```python
from build123d import *

# Parameters (mm, degrees)
F3_T      = -3.175
F5_DEPTH  = 31.75
F7_DEPTH  = 31.75
F9_DEPTH  = 31.75
F10_R     = 12.7
F11_DEPTH = 25.4
F12_W     = 12.7
F12_H     = 6.35
F13_DEPTH = 7.62
F15_DEPTH = 6.35
F16_R     = 6.35
F17_DEPTH = 25.4


with BuildPart() as f2:
    # F0 (on Front) → F2 (revolve)
    with BuildSketch(Plane.XZ):
        Polygon((-34.925, 0), (0, 0), (0, 34.925), (-47.625, 34.925), align=None)
    revolve(axis=Axis((0, 0, 24.3954025209), (0, 0, 1)))

    # F3
    f3_openings = [f2.faces().sort_by_distance(p)[0] for p in [
        (0, 0, 34.925),
    ]]
    offset(amount=F3_T, openings=f3_openings)

    # F4 (on face) → F5 (join)
    with BuildSketch(Plane(origin=(0, 0, 0), x_dir=(1, 0, 0), z_dir=(0, 0, -1))):
        with BuildLine():
            Line((-32.8328621344, 11.90625), (-11.90625, 11.90625))
            Line((-11.90625, 11.90625), (-11.90625, 32.8328621344))
            ThreePointArc((-11.90625, 32.8328621344), (-13.5101727919, 32.2060686227), (-15.08125, 31.5009765474))
            Line((-15.08125, 31.5009765474), (-15.08125, 15.08125))
            Line((-15.08125, 15.08125), (-31.5009765474, 15.08125))
            ThreePointArc((-31.5009765474, 15.08125), (-32.2060686227, 13.5101727919), (-32.8328621344, 11.90625))
        make_face()
        with BuildLine():
            Line((-11.90625, -32.8328621344), (-11.90625, -11.90625))
            Line((-11.90625, -11.90625), (-32.8328621344, -11.90625))
            ThreePointArc((-32.8328621344, -11.90625), (-32.2060686227, -13.5101727919), (-31.5009765474, -15.08125))
            Line((-31.5009765474, -15.08125), (-15.08125, -15.08125))
            Line((-15.08125, -15.08125), (-15.08125, -31.5009765474))
            ThreePointArc((-15.08125, -31.5009765474), (-13.5101727919, -32.2060686227), (-11.90625, -32.8328621344))
        make_face()
        with BuildLine():
            Line((32.8328621344, -11.90625), (11.90625, -11.90625))
            Line((11.90625, -11.90625), (11.90625, -32.8328621344))
            ThreePointArc((11.90625, -32.8328621344), (13.5101727919, -32.2060686227), (15.08125, -31.5009765474))
            Line((15.08125, -31.5009765474), (15.08125, -15.08125))
            Line((15.08125, -15.08125), (31.5009765474, -15.08125))
            ThreePointArc((31.5009765474, -15.08125), (32.2060686227, -13.5101727919), (32.8328621344, -11.90625))
        make_face()
        with BuildLine():
            Line((11.90625, 32.8328621344), (11.90625, 11.90625))
            Line((11.90625, 11.90625), (32.8328621344, 11.90625))
            ThreePointArc((32.8328621344, 11.90625), (32.2060686227, 13.5101727919), (31.5009765474, 15.08125))
            Line((31.5009765474, 15.08125), (15.08125, 15.08125))
            Line((15.08125, 15.08125), (15.08125, 31.5009765474))
            ThreePointArc((15.08125, 31.5009765474), (13.5101727919, 32.2060686227), (11.90625, 32.8328621344))
        make_face()
    extrude(amount=F5_DEPTH)

    # F6 (on face) → F7 (cut, through all)
    with BuildSketch(Plane.XY.offset(34.925)):
        Polygon((15.7154482119, 51.6364726961), (0, 0), (51.6364726961, 15.7154482119), (33.675960454, 33.675960454), align=None)
    extrude(amount=-F7_DEPTH, mode=Mode.SUBTRACT)

    # F8 (on face) → F9 (cut, through all)
    with BuildSketch(Plane.XY.offset(34.925)):
        with BuildLine():
            Line((-27.3165777812, 39.0121161093), (0, 0))
            Line((0, 0), (0, 47.625))
            ThreePointArc((0, 47.625), (-14.3211137014, 45.4207697794), (-27.3165777812, 39.0121161093))
        make_face()
        with BuildLine():
            Line((-39.0121161093, -27.3165777812), (0, 0))
            Line((0, 0), (-39.0121161093, 27.3165777812))
            ThreePointArc((-39.0121161093, 27.3165777812), (-47.625, 0), (-39.0121161093, -27.3165777812))
        make_face()
        with BuildLine():
            Line((27.3165777812, -39.0121161093), (0, 0))
            Line((0, 0), (-27.3165777812, -39.0121161093))
            ThreePointArc((-27.3165777812, -39.0121161093), (0, -47.625), (27.3165777812, -39.0121161093))
        make_face()
        with BuildLine():
            Line((47.625, 0), (0, 0))
            Line((0, 0), (39.0121161093, -27.3165777812))
            ThreePointArc((39.0121161093, -27.3165777812), (45.4207697794, -14.3211137014), (47.625, 0))
        make_face()
    extrude(amount=-F9_DEPTH, mode=Mode.SUBTRACT)

    # F10 (on face) → F11 (cut)
    with BuildSketch(Plane.XY.offset(3.175)):
        Circle(F10_R)
    extrude(amount=-F11_DEPTH, mode=Mode.SUBTRACT)

    # F12 (on face) → F13 (join)
    with BuildSketch(Plane.YZ.offset(15.08125)):
        with Locations((23.2911132737, -15.875)):
            Rectangle(F12_W, F12_H)
    extrude(amount=F13_DEPTH)

    # F14 (on face) → F15 (cut, through all)
    with BuildSketch(Plane(origin=(0, 0, -19.05), x_dir=(1, 0, 0), z_dir=(0, 0, -1))):
        with BuildLine():
            Line((16.1188345795, -28.8882274593), (20.7059307299, -22.1824388165))
            ThreePointArc((20.7059307299, -22.1824388165), (20.8007868478, -19.6961173416), (18.5999628156, -18.5354426503))
            Line((18.5999628156, -18.5354426503), (15.08125, -18.5354426503))
            Line((15.08125, -18.5354426503), (15.08125, -29.6411132737))
            Line((15.08125, -29.6411132737), (15.885964036, -29.6411132737))
            ThreePointArc((15.885964036, -29.6411132737), (15.9455112052, -29.2470746527), (16.1188345795, -28.8882274593))
        make_face()
        with BuildLine():
            ThreePointArc((19.52625, -16.9411132737), (21.7713140303, -17.8710492434), (22.70125, -20.1161132737))
            Line((22.70125, -20.1161132737), (22.70125, -16.9411132737))
            Line((22.70125, -16.9411132737), (19.52625, -16.9411132737))
        make_face()
        with BuildLine():
            Line((22.1467963251, -22.8878208585), (17.527205209, -29.6411132737))
            Line((17.527205209, -29.6411132737), (22.70125, -29.6411132737))
            Line((22.70125, -29.6411132737), (22.70125, -21.0952355863))
            ThreePointArc((22.70125, -21.0952355863), (22.5594710257, -22.0334227792), (22.1467963251, -22.8878208585))
        make_face()
    extrude(amount=-F15_DEPTH, mode=Mode.SUBTRACT)

    # F16 (on face) → F17 (cut)
    with BuildSketch(Plane.XY.offset(3.175)):
        with Locations((-24.3955454545, 0)):
            Circle(F16_R)
        with Locations((0, -24.3955454545)):
            Circle(F16_R)
        with Locations((24.3955454545, 0)):
            Circle(F16_R)
        with Locations((0, 24.3955454545)):
            Circle(F16_R)
    extrude(amount=-F17_DEPTH, mode=Mode.SUBTRACT)


solid = f2.part
```
Read the model definition and answer for the solid it produces. Units are mm, in the model's axes. A direction names the side the tool comes from. Coordinates: 2 decimals unless noted, no trailing zeros. Order: outer loops, then holes, each group sorted by start corner. A loop starts at its lowest first (then second) coordinate and runs counter-clockwise, first axis right, second up. Notation, with made-up numbers: (61, 84) - (95, 84) arc R20 ccw to (95, 112) - close; hole circle Ø4 at (-1, 41.25). An arc over 180 degrees is marked (long way). Answer as a JSON object with one key per item and string values. Group by question number.
Item 1: Section A-A (z = -21.5) is taken. Give the vertices of the cut face in (x, y) (3 decimals).
Item 2: Consider probe 1 along Y at (x, z) = (-25, -27.5); probe 2 along Y at (x, z) = (0, 1.2); probe 3 along Y at (x, z) = (0, 2). Determine where each line is inside the solid, lowest interval first. Write a range as from..to.
Item 3: A tool of negligible diameter and unlimited length cuts with its end or side. For faces 1 (the face through (13.488, 32.215, -15.653)), 2 (the face through (21.7, 17.8, -15.9)), 3 (the face through (32.871, -23.017, 19.124)), 4 (the face through (-23, 15.081, -16)), 5 (the face through (15.081, -23, -16)), from which of +Z, -Z, +X, -X, +Y, -Y can it reach the whole face along a straight path? Write none if from no direction.
Item 4: Flat-ended cylindrical pins translate along their axes: P1, Ø10.5, axis at x = -22.5, z = -13.5, coming from the -Y side; P2, Ø16.5, axis at y = 26.5, z = -20.5, coming from the +X side; P3, Ø12, axis at y = -6.5, z = -5.5, coming from the -X side; P4, Ø4, axis at x = -9.5, z = -3.5, coming from the +Y side. Find the tip coordinate at first contact, or state that the pin passes through.
Item 5: Section C-C (z = 9.5) is taken. Give the vertices of the cut face in (x, y).
Item 6: Section B-B (z = 21.5) is taken. Give the vertices of the cut face in (x, y).
Item 7: The mould has two halves that part along X. Classify faces 6 (the face through (38.39, 11.684, 19.124)), 7 (the face through (-11.906, -22, -16)), 8 (the face through (32.197, 13.532, -15.653)), 9 (the face through (-23, -15.081, -16)): +X half, -X half, draft (parallel to the pull), parting line (faces both ways), or undercut.
Results are:
{
 "1": {"outline": "(-32.833, -11.906) arc R34.925 ccw to (-31.501, -15.081) - (-15.081, -15.081) - (-15.081, -31.501) arc R34.925 ccw to (-11.906, -32.833) - (-11.906, -11.906) - close; (-32.833, 11.906) - (-11.906, 11.906) - (-11.906, 32.833) arc R34.925 ccw to (-15.081, 31.501) - (-15.081, 15.081) - (-31.501, 15.081) arc R34.925 ccw to start; (11.906, -32.833) arc R34.925 ccw to (15.081, -31.501) - (15.081, -15.081) - (31.501, -15.081) arc R34.925 ccw to (32.833, -11.906) - (11.906, -11.906) - close; (11.906, 11.906) - (32.833, 11.906) arc R34.925 ccw to (31.501, 15.081) - (15.081, 15.081) - (15.081, 31.501) arc R34.925 ccw to (11.906, 32.833) - close"},
 "2": {"probe 1": "y = -15.08..-11.91, 11.91..15.08", "probe 2": "y = -35.36..-30.75, -18.05..-12.7, 12.7..18.05, 30.75..35.36", "probe 3": "y = -35.65..-30.75, -18.05..-12.7, 12.7..18.05, 30.75..35.65"},
 "3": {"face 1": "-Z, +X, +Y", "face 2": "-Z, +X", "face 3": "+Z, +X, +Y", "face 4": "-Z, -X, +Y", "face 5": "-Z, +X, -Y"},
 "4": {"P1": "stops at y = -15.08", "P2": "stops at x = 22.7", "P3": "stops at x = -34.69", "P4": "passes through"},
 "5": {"outline": "(-31.44, -22.01) arc R38.38 ccw to (-22.01, -31.44) - (-20.08, -28.67) arc R35 cw to (-28.67, -20.08) - close; (-31.44, 22.01) - (-28.67, 20.08) arc R35 cw to (-20.08, 28.67) - (-22.01, 31.44) arc R38.38 ccw to start; (0, 35) arc R35 cw to (10.19, 33.48) - (11.17, 36.72) arc R38.38 ccw to (0, 38.38) - close; (20.08, -28.67) - (22.01, -31.44) arc R38.38 ccw to (31.44, -22.01) - (28.67, -20.08) arc R35 cw to start; (33.48, 10.19) arc R35 cw to (35, 0) - (38.38, 0) arc R38.38 ccw to (36.72, 11.17) - close"},
 "6": {"outline": "(-35.01, -24.52) arc R42.74 ccw to (-24.52, -35.01) - (-22.58, -32.25) arc R39.36 cw to (-32.25, -22.58) - close; (-35.01, 24.52) - (-32.25, 22.58) arc R39.36 cw to (-22.58, 32.25) - (-24.52, 35.01) arc R42.74 ccw to start; (0, 39.36) arc R39.36 cw to (11.46, 37.66) - (12.45, 40.89) arc R42.74 ccw to (0, 42.74) - close; (22.58, -32.25) - (24.52, -35.01) arc R42.74 ccw to (35.01, -24.52) - (32.25, -22.58) arc R39.36 cw to start; (37.66, 11.46) arc R39.36 cw to (39.36, 0) - (42.74, 0) arc R42.74 ccw to (40.89, 12.45) - close"},
 "7": {"face 6": "-X half", "face 7": "undercut", "face 8": "+X half", "face 9": "draft"}
}
